```python
from build123d import *

# Parameters (mm, degrees)
BOSS_EXTRUDE1_DEPTH     = 40
BOSS_EXTRUDE2_START     = 30
SKETCH2_R               = 1.25
BOSS_EXTRUDE2_DEPTH     = 10
CUT_EXTRUDE1_START      = -30
SKETCH3_W               = 5
SKETCH3_H               = 5
CUT_EXTRUDE1_DEPTH      = 10
CUT_EXTRUDE2_DEPTH      = 95.472218138
CUT_EXTRUDE2_DEPTH_BACK = 95.472218138
SKETCH4_R               = 1.25
FILLET1_R               = 2.5


with BuildPart() as part:
    # Sketch1 → Boss-Extrude1 (new, symmetric)
    with BuildSketch(Plane.XY):
        Polygon((0, 0), (85, 0), (85, 10), (80, 10), (80, 5), (0, 5), align=None)
    extrude(amount=BOSS_EXTRUDE1_DEPTH, both=True)

    # Sketch2 → Boss-Extrude2 (add)
    with BuildSketch(Plane.XY.offset(BOSS_EXTRUDE2_START)):
        with BuildLine():
            Line((0, 5), (-2.5, 5))
            ThreePointArc((-2.5, 5), (-5, 2.5), (-2.5, 0))
            Line((-2.5, 0), (0, 0))
            Line((0, 0), (0, 5))
        make_face()
        with Locations((-2.5, 2.5)):
            Circle(SKETCH2_R, mode=Mode.SUBTRACT)
    boss_extrude2 = extrude(amount=BOSS_EXTRUDE2_DEPTH)

    # Mirror2: Boss-Extrude2 across plane
    add(boss_extrude2.mirror(Plane.XY))

    # Sketch3 → Cut-Extrude1 (cut)
    with BuildSketch(Plane.XY.offset(CUT_EXTRUDE1_START)):
        with Locations((82.5, 7.5)):
            Rectangle(SKETCH3_W, SKETCH3_H)
    cut_extrude1 = extrude(amount=-CUT_EXTRUDE1_DEPTH, mode=Mode.SUBTRACT)

    # Mirror3: Cut-Extrude1 across plane
    add(cut_extrude1.mirror(Plane.XY), mode=Mode.SUBTRACT)

    # Sketch4 → Cut-Extrude2 (cut, two sides: drawn at the far end of the back side and taken through both)
    with BuildSketch(Plane.XY.offset(-CUT_EXTRUDE2_DEPTH_BACK)):
        with Locations((82.5, 7.5)):
            Circle(SKETCH4_R)
    extrude(amount=CUT_EXTRUDE2_DEPTH + CUT_EXTRUDE2_DEPTH_BACK, mode=Mode.SUBTRACT)

    # Fillet1
    fillet1_edges = [part.edges().sort_by_distance(p)[0] for p in [
        (80, 10, 0),
        (85, 10, 0),
    ]]
    fillet(fillet1_edges, radius=FILLET1_R - 0.0001)  # a hair under: the kernel refuses the full size


solid = part.part
```
Geometry check sheet. Reference: the model listing, model coordinates, mm. A direction names the side the tool comes from. Coordinates: 2 decimals unless noted, no trailing zeros. Order: outer loops, then holes, each group sorted by start corner. A loop starts at its lowest first (then second) coordinate and runs counter-clockwise, first axis right, second up. Notation, with made-up numbers: (-25, -30) - (10, -30) arc R12 ccw to (10, -10) - close; hole circle Ø5 at (3.5, 5). An arc over 180 degrees is marked (long way). Use one line per item in the form item = value.
1. Access from +Z, -Z, +X, -X, +Y, -Y to the whole of each face (thin tool, end or side, straight path). Record for faces 1 (the face through (80, 6, 0)), 2 (the face through (81, 7, 30)), 3 (the face through (-2, 4, 30)), 4 (the face through (81, 7, -30)).
Here are the results:
face_1 = +Z, -Z, -X, +Y
face_2 = +Z, +X, -X, +Y
face_3 = -X, +Y, -Y
face_4 = -Z, +X, -X, +Y
2. Gauge pin test, flat ends, axial feed: pin 1 (6 mm diameter, centred on y = 5, z = 9.5, fed in from -X); pin 2 (0.8 mm diameter, centred on y = 7, z = -5, fed in from -X); pin 3 (3 mm diameter, centred on x = -2.5, y = 2.5, fed in from -Z); pin 4 (5 mm diameter, centred on x = 50, z = -24, fed in from +Y). Record the tip position at first contact, or that the pin passes through.
Here are the results:
pin_1 = 0
pin_2 = 80
pin_3 = -40
pin_4 = 5
3. Section check B-B (x = 76). Record the boundary of the cut face in (y, z), then the cut area to 3 significant figures.
Here are the results:
outline = (0, -40) - (5, -40) - (5, 40) - (0, 40) - close
area = 400 mm²
4. Draft check along Y on faces 5 (the face through (-1.31, 2.88, -34.93)), 6 (the face through (-1.31, 2.88, 34.93)), 7 (the face through (39, 3, -40)), 8 (the face through (84.287, 9.248, 0.42)). Enter one of: pulls with the +Y half, pulls with the -Y half, needs draft (parallel to the pull), parting line crosses it, or undercut.
Here are the results:
face_5 = undercut
face_6 = undercut
face_7 = needs draft
face_8 = pulls with the +Y half
5. Scan lines: line 1 (X direction, y = 7.5, z = 15.5); line 2 (Y direction, x = 47.5, z = -26); line 3 (X direction, y = 3.75, z = 20.5). Record each from-to range of solid material in increasing order.
Here are the results:
line_1 = 80 to 81.25, 83.75 to 85
line_2 = 0 to 5
line_3 = 0 to 85
